from build123d import *

# Parameters (mm, degrees)
F0_R     = 10
F1_DEPTH = 20


with BuildPart() as f1:
    # F0 (on Right) → F1 (new body)
    with BuildSketch(Plane.YZ):
        with BuildLine():
            Line((0, 13.228757), (0, 5))
            ThreePointArc((0, 5), (5, 0), (0, -5))
            Line((0, -5), (0, -13.228757))
            Line((0, -13.228757), (4.114378, -13.228757))
            Line((4.114378, -13.228757), (4.114378, -9.114378))
            ThreePointArc((4.114378, -9.114378), (6.516361, -7.585317), (8.390026, -5.441274))
            Line((8.390026, -5.441274), (87.009619, -7.5))
            ThreePointArc((87.009619, -7.5), (115, 0), (87.009619, 7.5))
            Line((87.009619, 7.5), (8.390026, 5.441274))
            ThreePointArc((8.390026, 5.441274), (6.516361, 7.585317), (4.114378, 9.114378))
            Line((4.114378, 9.114378), (4.114378, 13.228757))
            Line((4.114378, 13.228757), (0, 13.228757))
        make_face()
        with Locations((100, 0)):
            Circle(F0_R, mode=Mode.SUBTRACT)
        with BuildLine():
            ThreePointArc((0, -5), (-5, 0), (0, 5))
            Line((0, 5), (0, 13.228757))
            Line((0, 13.228757), (-4.114378, 13.228757))
            Line((-4.114378, 13.228757), (-4.114378, 9.114378))
            ThreePointArc((-4.114378, 9.114378), (-10, 0), (-4.114378, -9.114378))
            Line((-4.114378, -9.114378), (-4.114378, -13.228757))
            Line((-4.114378, -13.228757), (0, -13.228757))
            Line((0, -13.228757), (0, -5))
        make_face()
    extrude(amount=F1_DEPTH)


solid = f1.part
For this review, take the finished solid that the model builds, in its own axes (mm). A direction names the side the tool comes from. Give positions to 0.01 mm unless a question says otherwise; leave off trailing zeros. Loops run counter-clockwise (first coordinate to the right, second up) from the corner with the lowest first, then second, coordinate; pieces in that order, holes last. Notation, with made-up numbers: (-15, 19) -> (39, 19) arc R24 cw to (39, 45) -> close; hole circle Ø5 at (-15.5, 79.25). An arc over 180 degrees is marked (long way). One line per question, with ' | ' between items.
1) For faces 1 (the flat face through (10, -4.114, 11)), 2 (the flat face through (10, -4.114, -11)), 3 (the cylindrical face through (10, 6, -8)), 4 (the flat face through (10, 4.114, 11)), list the 3-axis set-ups (+Z, -Z, +X, -X, +Y, -Y) from which the entire face can be reached by the end or side of a thin tool; tool diameter is ignored.
Resolved:
face 1: +Z, +X, -X, -Y | face 2: -Z, +X, -X, -Y | face 3: -Z, +X, -X | face 4: +Z, +X, -X
2) Insertion check: pin 1 Ø9 at (x, y) = (6, -0.5) entering from -Z; pin 2 Ø1.5 at (x, z) = (14.5, 3) entering from -Y; pin 3 Ø3.5 at (x, z) = (9.5, 11) entering from -Y. Each pin has a flat end and moves straight along its axis. Give the tip position at first contact, or say it passes through.
Resolved:
pin 1: stops at z = -13.23 | pin 2: stops at y = -9.74 | pin 3: stops at y = -4.11
3) We need section C-C (z = -3). Write out the cut boundary in (x, y), plus the area to 3 significant figures.
Resolved:
outline: (0, -9.54) -> (20, -9.54) -> (20, -4) -> (0, -4) -> close; (0, 4) -> (20, 4) -> (20, 90.46) -> (0, 90.46) -> close; (0, 109.54) -> (20, 109.54) -> (20, 114.7) -> (0, 114.7) -> close | area: 1,940 mm2
4) We need section B-B (y = 100). Write out the cut boundary in (x, z), plus the area to 3 significant figures.
Resolved:
outline: (0, -15) -> (20, -15) -> (20, -10) -> (0, -10) -> close; (0, 10) -> (20, 10) -> (20, 15) -> (0, 15) -> close | area: 200 mm2
5) We need section D-D (z = 11.75). Write out the cut boundary in (x, y).
Resolved:
outline: (0, -4.11) -> (20, -4.11) -> (20, 4.11) -> (0, 4.11) -> close; (0, 90.68) -> (20, 90.68) -> (20, 109.32) -> (0, 109.32) -> close
6) The part is to be moulded in two halves that separate along Z. For faces 5 (the flat face through (10, 0, -13.229)), 6 (the cylindrical face through (10, 90, 0)), 7 (the cylindrical face through (10, 3, 4)), 8 (the flat face through (10, 4.114, -11)), say which applies: +Z half, -Z half, draft (parallel to the pull), parting line (faces both ways), or undercut.
Resolved:
face 5: -Z half | face 6: undercut | face 7: undercut | face 8: draft
7) To check wall thickness, follow probe 1 along Y at (x, z) = (12, -9); probe 2 along Y at (x, z) = (19.25, -4.5); probe 3 along Y at (x, z) = (16, -10.25). State the ranges of each line that lie inside material, in increasing order.
Resolved:
probe 1: y = -4.36 to 4.36, 88 to 95.64, 104.36 to 112 | probe 2: y = -8.93 to -2.18, 2.18 to 91.07, 108.93 to 114.31 | probe 3: y = -4.11 to 4.11, 89.05 to 110.95
8) We need section A-A (x = 5.5). Write out the cut boundary in (y, z).
Resolved:
outline: (-4.11, -13.23) -> (4.11, -13.23) -> (4.11, -9.11) arc R10 ccw to (8.39, -5.44) -> (87.01, -7.5) arc R15 ccw (long way) to (87.01, 7.5) -> (8.39, 5.44) arc R10 ccw to (4.11, 9.11) -> (4.11, 13.23) -> (-4.11, 13.23) -> (-4.11, 9.11) arc R10 ccw to (-4.11, -9.11) -> close; hole circle Ø10 at (0, 0); hole circle Ø20 at (100, 0)
